```python
from build123d import *

# Parameters (mm, degrees)
SALIENTE_EXTRUIR1_DEPTH = 80
CROQUIS3_R              = 1.5
CROQUIS3_R_2            = 3.6
CORTAR_EXTRUIR2_DEPTH   = 155.44497402
CROQUIS4_R              = 3.75
CORTAR_EXTRUIR3_DEPTH   = 80
CROQUIS5_R              = 7.565
CROQUIS5_R_2            = 8.5
CROQUIS5_R_3            = 4
CROQUIS5_R_4            = 3.75
CORTAR_EXTRUIR4_DEPTH   = 80
SALIENTE_EXTRUIR2_DEPTH = 1.5
SALIENTE_EXTRUIR4_DEPTH = 1.5


with BuildPart() as part:
    # Croquis1 → Saliente-Extruir1 (new body)
    with BuildSketch(Plane.XY):
        with BuildLine():
            Line((0, 0), (0, 28))
            ThreePointArc((0, 28), (0.146446609, 28.353553391), (0.5, 28.5))
            Line((0.5, 28.5), (128.5, 28.5))
            ThreePointArc((128.5, 28.5), (128.853553391, 28.353553391), (129, 28))
            Line((129, 28), (129, 0))
            Line((129, 0), (127.5, 0))
            Line((127.5, 0), (127.5, 26.5))
            ThreePointArc((127.5, 26.5), (127.353553391, 26.853553391), (127, 27))
            Line((127, 27), (2, 27))
            ThreePointArc((2, 27), (1.646446609, 26.853553391), (1.5, 26.5))
            Line((1.5, 26.5), (1.5, 0))
            Line((1.5, 0), (0, 0))
        make_face()
    extrude(amount=SALIENTE_EXTRUIR1_DEPTH)

    # Croquis3 → Cortar-Extruir2 (cut, through all)
    with BuildSketch(Plane(origin=(0, 0, 0), x_dir=(0, 0, -1), z_dir=(1, 0, 0))):
        with Locations(Location((-48.28, 3.65, 0), (0, 0, 270))):
            Circle(CROQUIS3_R)
        with Locations(Location((-65.8, 12.85, 0), (0, 0, 270))):
            Circle(CROQUIS3_R)
        with Locations(Location((-63.75, 6.26, 0), (0, 0, 270))):
            Circle(CROQUIS3_R_2)
        with Locations(Location((-31.72, 3.65, 0), (0, 0, 180))):
            Circle(CROQUIS3_R)
        with Locations(Location((-16.25, 6.26, 0), (0, 0, 180))):
            Circle(CROQUIS3_R_2)
        with Locations(Location((-14.2, 12.85, 0), (0, 0, 180))):
            Circle(CROQUIS3_R)
    extrude(amount=CORTAR_EXTRUIR2_DEPTH, mode=Mode.SUBTRACT)

    # Croquis4 → Cortar-Extruir3 (cut)
    with BuildSketch(Plane(origin=(0, 0, 0), x_dir=(0, 0, -1), z_dir=(1, 0, 0))):
        with Locations(Location((-39.95, 22.7, 0), (0, 0, 270))):
            Circle(CROQUIS4_R)
        with Locations(Location((-24.95, 22.7, 0), (0, 0, 270))):
            Circle(CROQUIS4_R)
        with Locations(Location((-54.95, 22.7, 0), (0, 0, 270))):
            Circle(CROQUIS4_R)
    extrude(amount=CORTAR_EXTRUIR3_DEPTH, mode=Mode.SUBTRACT)

    # Croquis5 → Cortar-Extruir4 (cut)
    with BuildSketch(Plane(origin=(0, 0, 0), x_dir=(1, 0, 0), z_dir=(0, 1, 0))):
        with Locations((21.5, -65.92)):
            Circle(CROQUIS5_R)
        with Locations((64.5, 2)):
            Circle(CROQUIS5_R_2)
        with Locations((86.38, -40)):
            Circle(CROQUIS5_R_3)
        with Locations((64.5, -17.87)):
            Circle(CROQUIS5_R_3)
        with Locations((64.5, -62.13)):
            Circle(CROQUIS5_R_3)
        with Locations((107.5, -65.92)):
            Circle(CROQUIS5_R)
        with Locations((21.5, -14.08)):
            Circle(CROQUIS5_R)
        with Locations((107.5, -14.08)):
            Circle(CROQUIS5_R)
        with Locations(Location((5.5, -24.95, 0), (0, 0, 158.960530219))):
            Circle(CROQUIS5_R_4)
        with Locations(Location((5.5, -39.95, 0), (0, 0, 158.960530219))):
            Circle(CROQUIS5_R_4)
        with Locations(Location((5.5, -54.95, 0), (0, 0, 158.960530219))):
            Circle(CROQUIS5_R_4)
    extrude(amount=CORTAR_EXTRUIR4_DEPTH, mode=Mode.SUBTRACT)

    # Croquis6 → Saliente-Extruir2 (add)
    with BuildSketch(Plane.XY):
        Polygon((18.104253919, 27), (1.5, 10.395746081), (1.5, 27), align=None)
        Polygon((127.5, 27), (127.5, 10.395746081), (110.895746081, 27), align=None)
    extrude(amount=SALIENTE_EXTRUIR2_DEPTH)

    # Croquis7 → Saliente-Extruir4 (add)
    with BuildSketch(Plane.XY.offset(80)):
        Polygon((1.5, 27), (18.104253919, 27), (1.5, 10.395746081), align=None)
        Polygon((127.5, 27), (127.5, 10.395746081), (110.895746081, 27), align=None)
    extrude(amount=-SALIENTE_EXTRUIR4_DEPTH)


solid = part.part
```
Input: part model. Units: mm. Frame: model coordinates. A direction names the side the tool comes from. Round coordinates to 2 decimals unless told otherwise and drop trailing zeros. Loops run counter-clockwise (first coordinate to the right, second up) from the corner with the lowest first, then second, coordinate; pieces in that order, holes last. Notation, with made-up numbers: M 2.25,65 L 8.25,65 A12 ccw 8.25,77 Z; hole C 46.25,-11 d10. An arc over 180 degrees is marked long. Answer in a Markdown table with one row per item. Add a question column.
1. Set-up query: faces 1 (the face through (0.74, 25.464, 22.416)), 2 (the face through (119.314, 18.582, 79.26)), 3 (the face through (19.86, 27.74, 73.305)), 4 (the face through (65, 27, 39)). Return all of +Z, -Z, +X, -X, +Y, -Y with unobstructed straight access to the full face (end or side cutting, diameter ignored); none if empty.
2. Mould query, pull axis Y, two halves, no side actions, for faces 5 (the face through (119.314, 18.582, 0.74)), 6 (the face through (0.74, 3.58, 30.22)), 7 (the face through (114.488, 27.74, 16.977)). Classes: released by +Y, released by -Y, zero draft, split by the parting line, or undercut.
3. Ray query, probe 1 along Z at (x, y) = (21.5, 28.15) (3 decimals); probe 2 along X at (y, z) = (26, 59.5); probe 3 along Z at (x, y) = (1.05, 22.7). Return the intervals inside material, ascending.
4. Section A-A (x = 64.5). Output: boundary loops of the cut face in (y, z).
5. Contact query for flat-ended pins moving along their axis: pin 1 (2.5 mm diameter, centred on y = 3.65, z = 31.72, fed in from +X); pin 2 (8.5 mm diameter, centred on y = 6.26, z = 16.25, fed in from +X). Output: stop coordinate, or through.
6. Section C-C (y = 24.5). Output: boundary loops of the cut face in (x, z), and give its area (3 significant figures).
7. Section D-D (x = 86.38). Output: boundary loops of the cut face in (y, z).
8. Section B-B (z = 54.95). Output: boundary loops of the cut face in (x, y), and give its area (3 significant figures).
Values follow:
| question | item | result |
|---|---|---|
| 1 | face 1 | -X |
| 1 | face 2 | +Z, -Z, -Y |
| 1 | face 3 | +Y, -Y |
| 1 | face 4 | -Y |
| 2 | face 5 | released by -Y |
| 2 | face 6 | undercut |
| 2 | face 7 | zero draft |
| 3 | probe 1 | 0 to 6.515, 21.645 to 58.355, 73.485 to 80 |
| 3 | probe 2 | 0 to 1.5, 127.5 to 129 |
| 3 | probe 3 | 0 to 21.2, 28.7 to 36.2, 43.7 to 51.2, 58.7 to 80 |
| 4 | outline | M 27,6.5 L 28.5,6.5 L 28.5,13.87 L 27,13.87 Z; M 27,21.87 L 28.5,21.87 L 28.5,58.13 L 27,58.13 Z; M 27,66.13 L 28.5,66.13 L 28.5,80 L 27,80 Z |
| 5 | pin 1 | through |
| 5 | pin 2 | x = 129 |
| 6 | outline | M 0,0 L 15.6,0 L 15.6,1.5 L 1.5,1.5 L 1.5,21.66 L 0,21.66 Z; M 0,28.24 L 1.5,28.24 L 1.5,36.66 L 0,36.66 Z; M 0,43.24 L 1.5,43.24 L 1.5,51.66 L 0,51.66 Z; M 0,58.24 L 1.5,58.24 L 1.5,78.5 L 15.6,78.5 L 15.6,80 L 0,80 Z; M 113.4,0 L 129,0 L 129,80 L 113.4,80 L 113.4,78.5 L 127.5,78.5 L 127.5,1.5 L 113.4,1.5 Z |
| 6 | area | 295 mm^2 |
| 7 | outline | M 27,0 L 28.5,0 L 28.5,36 L 27,36 Z; M 27,44 L 28.5,44 L 28.5,80 L 27,80 Z |
| 8 | outline | M 0,0 L 1.5,0 L 1.5,18.95 L 0,18.95 Z; M 0,26.45 L 1.5,26.45 L 1.5,26.5 A0.5 cw 1.75,26.93 L 1.75,28.5 L 0.5,28.5 A0.5 ccw 0,28 Z; M 9.25,27 L 127,27 A0.5 cw 127.5,26.5 L 127.5,0 L 129,0 L 129,28 A0.5 ccw 128.5,28.5 L 9.25,28.5 Z |
| 8 | area | 252 mm^2 |
